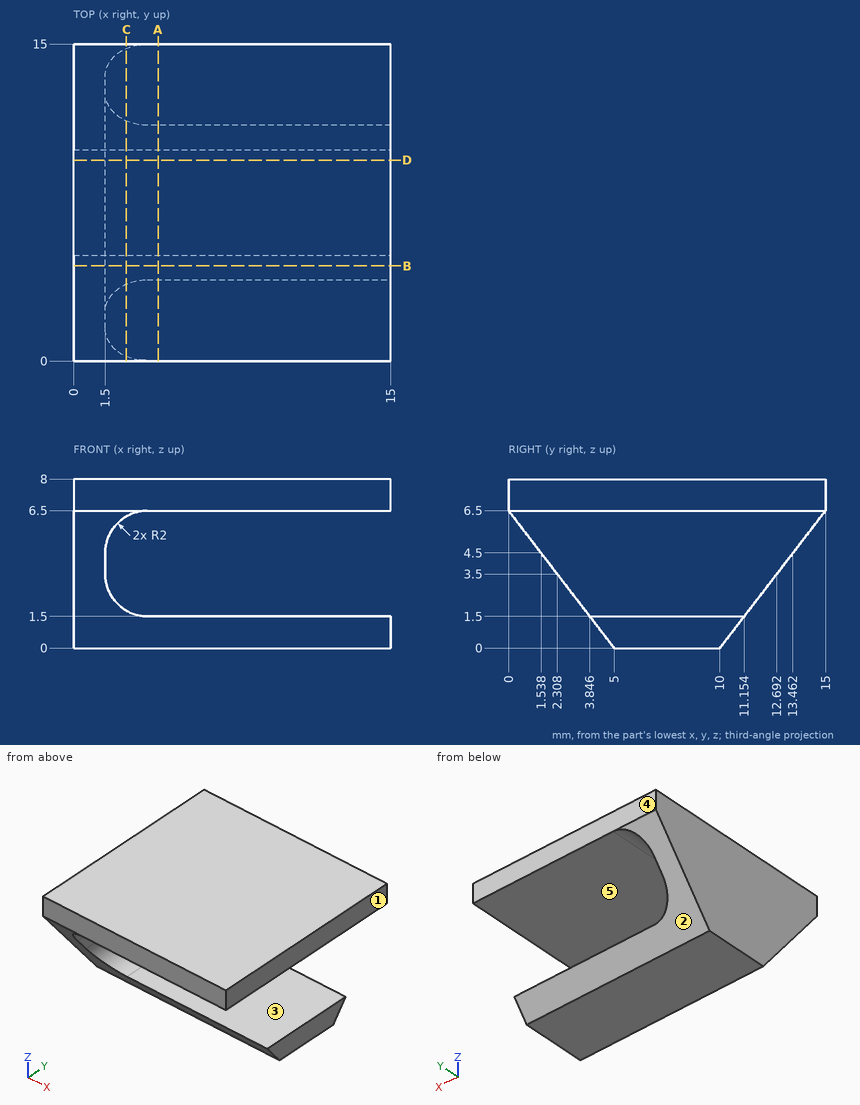
Verification items for this drawing (mm, ordinates from the low corner). A direction names the side the tool comes from. Give positions to 0.01 mm unless a question says otherwise; leave off trailing zeros. Write each loop counter-clockwise with the first axis right and the second up, starting at its lowest first coordinate (ties: lowest second). Pieces come first, ordered by that corner, then holes. Notation, with made-up numbers: (-5.5, 22.5) -> (37.5, 22.5) arc R21 ccw to (37.5, 45.5) -> close; hole circle Ø7 at (-13.5, 44). An arc over 180 degrees is marked (long way). Use CSV: the item, a comma, the result in double quotes.
(1) Sectioned sample at D-D (y = 9.5). Record the cut outline in (x, z).
Derived:
outline,"(0, 0) -> (15, 0) -> (15, 1.5) -> (3.5, 1.5) arc R2 cw to (1.5, 3.5) -> (1.5, 4.5) arc R2 cw to (3.5, 6.5) -> (15, 6.5) -> (15, 8) -> (0, 8) -> close"
(2) Sectioned sample at C-C (x = 2.5). Record the cut outline in (y, z).
Derived:
outline,"(0, 6.5) -> (0.21, 6.23) -> (14.79, 6.23) -> (15, 6.5) -> (15, 8) -> (0, 8) -> close; (3.64, 1.77) -> (5, 0) -> (10, 0) -> (11.36, 1.77) -> close"
(3) Sectioned sample at B-B (y = 4.5). Record the cut outline in (x, z).
Derived:
outline,"(0, 0.65) -> (15, 0.65) -> (15, 1.5) -> (3.5, 1.5) arc R2 cw to (1.5, 3.5) -> (1.5, 4.5) arc R2 cw to (3.5, 6.5) -> (15, 6.5) -> (15, 8) -> (0, 8) -> close"
(4) Material ranges on L1, parallel to Z at x = 5, y = 8.25; L2, parallel to Z at x = 14, y = 3; L3, parallel to Y at x = 1.5, z = 3, recorded low to high.
Derived:
L1,"z = 0 to 1.5, 6.5 to 8"
L2,"z = 6.5 to 8"
L3,"y = 2.69 to 12.31"
(5) Release check for a two-part mould opening along Z. For the marked faces 1, 2 and 3 record: +Z half, -Z half, draft (parallel to the pull), parting line (faces both ways), or undercut.
Derived:
face 1,"draft"
face 2,"-Z half"
face 3,"undercut"
(6) Set-up check for the marked faces 4 and 5: record each of +Z, -Z, +X, -X, +Y, -Y from which the full face is reachable in a straight line by a thin tool's end or side.
Derived:
face 4,"+Z, -Z, +X, -X, +Y"
face 5,"+X, +Y, -Y"
(7) Go/stop test with flat-tipped pins: pin 1 (2 mm diameter, centred on y = 1.5, z = 1.5, fed in from +X); pin 2 (1.1 mm diameter, centred on y = 9.5, z = 4, fed in from +X); pin 3 (3.5 mm diameter, centred on x = 7, y = 11, fed in from -Z). Record where each tip stops, or that it passes through.
Derived:
pin 1,"passes through"
pin 2,"stops at x = 1.5"
pin 3,"stops at z = 0"
(8) Sectioned sample at A-A (x = 4). Record the cut outline in (y, z).
Derived:
outline,"(0, 6.5) -> (15, 6.5) -> (15, 8) -> (0, 8) -> close; (3.85, 1.5) -> (5, 0) -> (10, 0) -> (11.15, 1.5) -> close"
